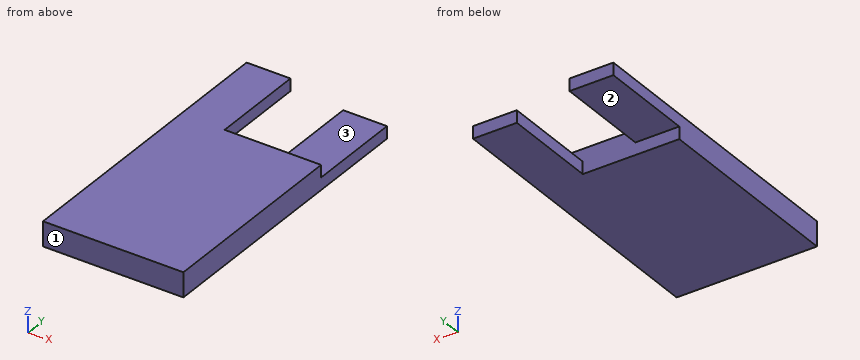
Autodesk Inventor part; units mm, degrees
ref_plane "YZ Plane" through (0, 0, 0) normal (1, 0, 0) x (0, 1, 0)
ref_plane "XZ Plane" through (0, 0, 0) normal (0, 1, 0) x (-1, 0, 0)
ref_plane "XY Plane" through (0, 0, 0) normal (0, 0, 1) x (1, 0, 0)
sketch "Sketch1" plane through (0, 0, 0) normal (0, 0, 1) x (1, 0, 0)
  line L0 (-4, 8.5) -> (4, 8.5)
  line L1 (4, 8.5) -> (4, -8.5)
  line L2 (4, -8.5) -> (-4, -8.5)
  line L3 (-4, -8.5) -> (-4, 8.5)
  line L4 (-4, 8.5) -> (4, -8.5) construction
  line L5 (4, 8.5) -> (-4, -8.5) construction
  point P0 (0, 0)
  dimension "d0" = 8
  dimension "d1" = 17
extrude "Extrusion1" add sketch "Sketch1" along normal blind 1.4
sketch "Sketch2" plane through (0, 0, 1.4) normal (0, 0, 1) x (1, 0, 0)
  line L0 (4, 8.5) -> (-4, 8.5)
  line L1 (-1.5, 8.5) -> (1.5, 8.5)
  line L2 (1.5, 8.5) -> (1.5, 3)
  line L3 (1.5, 3) -> (-1.5, 3)
  line L4 (-1.5, 3) -> (-1.5, 8.5)
  line L5 (4, -8.5) -> (4, 8.5)
  point P0 (0, 0)
  point P1 (1.5, 8.5)
  dimension "d4" = 3
  dimension "d5" = 5.5
  dimension "d6" = 2.5
extrude "Extrusion2" cut sketch "Sketch2" against normal blind 1.4
sketch "Sketch3" plane through (0, 0, 1.4) normal (0, 0, 1) x (1, 0, 0)
  line L0 (4, 8.5) -> (1.5, 8.5)
  line L1 (4, -8.5) -> (4, 8.5)
  line L2 (1.5, 8.5) -> (4, 8.5)
  line L3 (4, 8.5) -> (4, 3)
  line L4 (4, 3) -> (1.5, 3)
  line L5 (1.5, 3) -> (1.5, 8.5)
  point P0 (0, 0)
  dimension "d9" = 5.5
extrude "Extrusion3" cut sketch "Sketch3" against normal blind 0.7
sketch "Sketch4" plane through (0, 0, 0) normal (0, 0, -1) x (-1, 0, 0)
  line L0 (1.5, 3) -> (-1.5, 3)
  line L1 (4, 8.5) -> (4, -8.5)
  line L2 (1.5, 3) -> (4, 3)
  line L3 (4, 3) -> (4, 8.5)
  line L4 (4, 8.5) -> (1.5, 8.5)
  line L5 (1.5, 8.5) -> (1.5, 3)
  point P0 (0, 0)
extrude "Extrusion4" cut sketch "Sketch4" against normal blind 0.7
properties part number "Thermistor"
For this review, take the finished solid that the model builds, in its own axes (mm). Face numbers are marked on the shaded views. A direction names the side the tool comes from. Round coordinates to 2 decimals unless told otherwise and drop trailing zeros. Write each loop counter-clockwise with the first axis right and the second up, starting at its lowest first coordinate (ties: lowest second). Pieces come first, ordered by that corner, then holes. Notation, with made-up numbers: M 35.25,63 L 68.25,63 A32 ccw 68.25,96 Z; hole C 54.25,4 d7. An arc over 180 degrees is marked long. One line per item, written item: value. Start each with the question number.
(1) We need section C-C (x = 2). Give the boundary of the cut face in (y, z), and give its area (4 significant figures).
(2) We need section D-D (x = 0). Give the boundary of the cut face in (y, z).
(3) We need section B-B (z = 1.15). Give the boundary of the cut face in (x, y), and give its area (3 significant figures).
(4) Insertion check: pin 1 (2 mm diameter, centred on x = -3, y = 5, fed in from -Z); pin 2 (2 mm diameter, centred on x = 2, y = 6, fed in from +Z). Each pin has a flat end and moves straight along its axis. Give the tip position at first contact, or say it passes through.
(5) We need section A-A (y = 4.75). Give the boundary of the cut face in (x, z), and give its area (3 significant figures).
(6) Machinability: for the marked faces 1, 2 and 3, which of the approach directions +Z, -Z, +X, -X, +Y, -Y give a long, thin tool a straight path to every point of the face, cutting with its end or side? Answer none if there is none.
(7) Wall thickness on line 1 (Y direction, x = -2.75, z = 0.4); line 2 (X direction, y = 6, z = 0.55); line 3 (Z direction, x = 3, y = 4.5): over which ranges is each line inside the solid? List them lowest first.
Result:
1. outline: M -8.5,0 L 8.5,0 L 8.5,0.7 L 3,0.7 L 3,1.4 L -8.5,1.4 Z
1. area: 19.95 mm²
2. outline: M -8.5,0 L 3,0 L 3,1.4 L -8.5,1.4 Z
3. outline: M -4,-8.5 L 4,-8.5 L 4,3 L -1.5,3 L -1.5,8.5 L -4,8.5 Z
3. area: 106 mm²
4. pin 1: z = 0.7
4. pin 2: z = 0.7
5. outline: M -4,0.7 L -1.5,0.7 L -1.5,1.4 L -4,1.4 Z; M 1.5,0 L 4,0 L 4,0.7 L 1.5,0.7 Z
5. area: 3.50 mm²
6. face 1: +Z, -Z, +X, -X, -Y
6. face 2: -Z, -X, +Y
6. face 3: +Z, +X, +Y
7. line 1: -8.5 to 3
7. line 2: 1.5 to 4
7. line 3: 0 to 0.7
